from build123d import *

# Parameters (mm, degrees)
SKETCH1_R           = 10
BOSS_EXTRUDE1_DEPTH = 35
SKETCH3_R           = 4
CUT_EXTRUDE2_DEPTH  = 15
CUT_EXTRUDE1_DEPTH  = 15


with BuildPart() as part:
    # Sketch1 → Boss-Extrude1 (new body)
    with BuildSketch(Plane(origin=(0, 0, 0), x_dir=(1, 0, 0), z_dir=(0, 1, 0))):
        with Locations(Location((0, 0, 0), (0, 0, 270))):
            Circle(SKETCH1_R)
    extrude(amount=BOSS_EXTRUDE1_DEPTH)

    # Sketch3 → Cut-Extrude2 (cut)
    with BuildSketch(Plane.XZ):
        with Locations(Location((0, 0, 0), (0, 0, 270))):
            Circle(SKETCH3_R)
    extrude(amount=-CUT_EXTRUDE2_DEPTH, mode=Mode.SUBTRACT)

    # Sketch2 → Cut-Extrude1 (cut)
    with BuildSketch(Plane(origin=(0, 35, 0), x_dir=(1, 0, 0), z_dir=(0, 1, 0))):
        with BuildLine():
            Line((1.5, 2), (-1.5, 2))
            ThreePointArc((-1.5, 2), (-1.118033989, -2.236067977), (2.5, 0))
            ThreePointArc((2.5, 0), (2.236067977, 1.118033989), (1.5, 2))
        make_face()
    extrude(amount=-CUT_EXTRUDE1_DEPTH, mode=Mode.SUBTRACT)


solid = part.part
Source: CAD feature listing. Evaluate the final solid. Frame: model axes, mm. A direction names the side the tool comes from. Coordinates: 2 decimals unless noted, no trailing zeros. Loops run counter-clockwise (first coordinate to the right, second up) from the corner with the lowest first, then second, coordinate; pieces in that order, holes last. Notation, with made-up numbers: M 20.25,83 L 61.25,83 A24 cw 61.25,102 Z; hole C 88.5,76 d4. An arc over 180 degrees is marked long. Answer in a Markdown table with one row per item.
Q1. Section B-B on y = 11.5. Return the cut outline in (x, z), plus the area to 3 significant figures.
Answers below:
| item | result |
|---|---|
| outline | C 0,0 d20; hole C 0,0 d8 |
| area | 264 mm^2 |
Q2. Ray query, probe 1 along X at (y, z) = (8.75, 0); probe 2 along X at (y, z) = (31.75, 0); probe 3 along Y at (x, z) = (-0.25, 0.25). Return the intervals inside material, ascending. Write a range as from..to.
Answers below:
| item | result |
|---|---|
| probe 1 | x = -10..-4, 4..10 |
| probe 2 | x = -10..-2.5, 2.5..10 |
| probe 3 | y = 15..20 |
Q3. Draft query along X for faces 4 (the cylindrical face through (-9.76, 17.26, -2.17)), 5 (the flat face through (0, 15, 0)), 6 (the flat face through (0.1, 0, 4.3)). Return one class per face: pulls with the +X half, pulls with the -X half, needs draft (parallel to the pull), parting line crosses it, or undercut.
Answers below:
| item | result |
|---|---|
| face 4 | parting line crosses it |
| face 5 | undercut |
| face 6 | needs draft |
Q4. Section D-D on y = 16. Return the cut outline in (x, z), plus the area to 3 significant figures.
Answers below:
| item | result |
|---|---|
| outline | C 0,0 d20 |
| area | 314 mm^2 |
Q5. Set-up query: faces 1 (the flat face through (0, 28, -2)), 2 (the flat face through (0.1, 35, -2.4)), 3 (the cylindrical face through (-3.905, 7.395, 0.867)). Return all of +Z, -Z, +X, -X, +Y, -Y with unobstructed straight access to the full face (end or side cutting, diameter ignored); none if empty.
Answers below:
| item | result |
|---|---|
| face 1 | +Y |
| face 2 | +Z, -Z, +X, -X, +Y |
| face 3 | -Y |
Q6. First-contact query: pin 1 (1.3 mm diameter, centred on x = 1, z = -0.5, fed in from +Y); pin 2 (5 mm diameter, centred on x = 4.5, y = 9.5, fed in from +Z); pin 3 (5 mm diameter, centred on y = 22, z = -3.5, fed in from +X). Flat tips, straight axial feed; report the tip coordinate or a pass-through.
Answers below:
| item | result |
|---|---|
| pin 1 | stops at y = 20 |
| pin 2 | stops at z = 9.8 |
| pin 3 | stops at x = 9.95 |
Q7. Section A-A on x = 0. Return the cut outline in (y, z), plus the area to 4 significant figures.
Answers below:
| item | result |
|---|---|
| outline | M 0,-10 L 35,-10 L 35,-2 L 20,-2 L 20,2.5 L 35,2.5 L 35,10 L 0,10 L 0,4 L 15,4 L 15,-4 L 0,-4 Z |
| area | 512.5 mm^2 |
Q8. Section C-C on z = -2.5. Return the cut outline in (x, y), plus the area to 3 significant figures.
Answers below:
| item | result |
|---|---|
| outline | M -9.68,0 L -3.12,0 L -3.12,15 L 3.12,15 L 3.12,0 L 9.68,0 L 9.68,35 L -9.68,35 Z |
| area | 584 mm^2 |
